Input: dimensioned drawing with shaded views. Units: mm. Origin: part minimum x, y, z. A direction names the side the tool comes from. Round coordinates to 2 decimals unless told otherwise and drop trailing zeros. Loops run counter-clockwise (first coordinate to the right, second up) from the corner with the lowest first, then second, coordinate; pieces in that order, holes last.
Item 1: Section query D-D on x = 9.5. Return loops of the section in (y, z), then the cut area to 3 significant figures.
Item 2: Section query A-A on x = 19.05. Return loops of the section in (y, z), then the cut area to 3 significant figures.
Item 3: Section query B-B on z = 34. Return loops of the section in (x, y).
Item 4: Ray query, L1, parallel to X at y = 19, z = 109.5; L2, parallel to Z at x = 36, y = 24.5; L3, parallel to Z at x = 11, y = 11. Return the intervals inside material, ascending.
Item 5: Section query C-C on y = 14.5. Return loops of the section in (x, z) (1 decimal), then the cut area to 3 significant figures.
Item 6: First-contact query: P1, Ø1.5, axis at y = 10.5, z = 118, coming from the +X side; P2, Ø2, axis at y = 10.5, z = 74.5, coming from the -X side; P3, Ø12, axis at x = 20.5, z = 73.5, coming from the +Y side. Flat tips, straight axial feed; report the tip coordinate or a pass-through.
Item 7: Access query for the marked faces 1 and 2. Directions: +Z, -Z, +X, -X, +Y, -Y. A direction counts if a zero-diameter tool reaches every point of the face in a straight line with its end or side. Return the directions, or none.
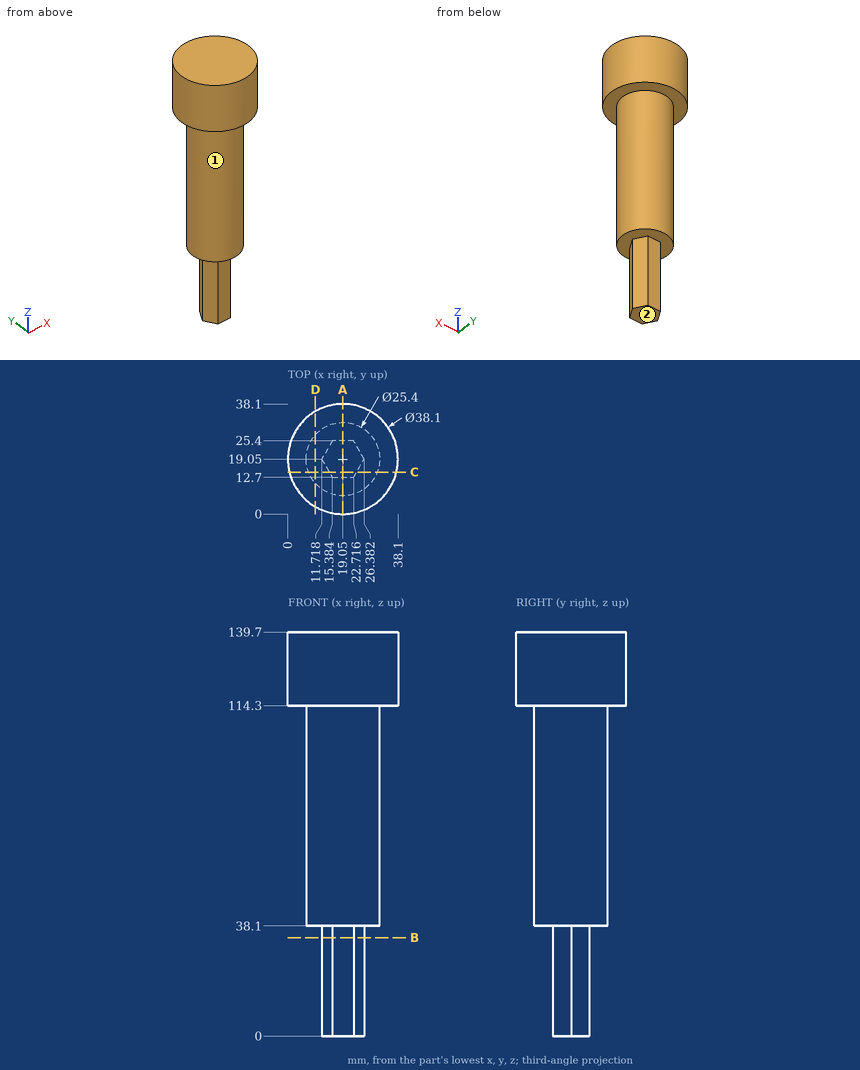
Data:
1. outline: (2.57, 114.3) - (10.68, 114.3) - (10.68, 38.1) - (27.42, 38.1) - (27.42, 114.3) - (35.53, 114.3) - (35.53, 139.7) - (2.57, 139.7) - close
1. area: 2,110 mm2
2. outline: (0, 114.3) - (6.35, 114.3) - (6.35, 38.1) - (12.7, 38.1) - (12.7, 0) - (25.4, 0) - (25.4, 38.1) - (31.75, 38.1) - (31.75, 114.3) - (38.1, 114.3) - (38.1, 139.7) - (0, 139.7) - close
2. area: 3,390 mm2
3. outline: (11.72, 19.05) - (15.38, 12.7) - (22.72, 12.7) - (26.38, 19.05) - (22.72, 25.4) - (15.38, 25.4) - close
4. L1: x = 6.35 to 31.75
4. L2: z = 114.3 to 139.7
4. L3: z = 38.1 to 139.7
5. outline: (0.6, 114.3) - (7.2, 114.3) - (7.2, 38.1) - (14.3, 38.1) - (14.3, 0) - (23.8, 0) - (23.8, 38.1) - (30.9, 38.1) - (30.9, 114.3) - (37.5, 114.3) - (37.5, 139.7) - (0.6, 139.7) - close
5. area: 3,110 mm2
6. P1: stops at x = 36.43
6. P2: stops at x = 8.84
6. P3: stops at y = 31.75
7. face 1: -Z
7. face 2: -Z, +X, -X, +Y, -Y
